from build123d import *

# Parameters (mm, degrees)
SKETCH1_R           = 0.575
SKETCH1_R_2         = 1.375
BOSS_EXTRUDE1_DEPTH = 1.2


with BuildPart() as part:
    # Sketch1 → Boss-Extrude1 (new body)
    with BuildSketch(Plane(origin=(0, 0, 0), x_dir=(1, 0, 0), z_dir=(0, 1, 0))):
        with BuildLine():
            Line((3, 0), (62, 0))
            ThreePointArc((62, 0), (64.121320344, 0.878679656), (65, 3))
            Line((65, 3), (65, 27))
            ThreePointArc((65, 27), (64.121320344, 29.121320344), (62, 30))
            Line((62, 30), (3, 30))
            ThreePointArc((3, 30), (0.878679656, 29.121320344), (0, 27))
            Line((0, 27), (0, 3))
            ThreePointArc((0, 3), (0.878679656, 0.878679656), (3, 0))
        make_face()
        with Locations((6.5, 27.85)):
            Circle(SKETCH1_R, mode=Mode.SUBTRACT)
        with Locations((9.236842105, 27.85)):
            Circle(SKETCH1_R, mode=Mode.SUBTRACT)
        with Locations((11.973684211, 27.85)):
            Circle(SKETCH1_R, mode=Mode.SUBTRACT)
        with Locations((14.710526316, 27.85)):
            Circle(SKETCH1_R, mode=Mode.SUBTRACT)
        with Locations((17.447368421, 27.85)):
            Circle(SKETCH1_R, mode=Mode.SUBTRACT)
        with Locations((20.184210526, 27.85)):
            Circle(SKETCH1_R, mode=Mode.SUBTRACT)
        with Locations((22.921052632, 27.85)):
            Circle(SKETCH1_R, mode=Mode.SUBTRACT)
        with Locations((25.657894737, 27.85)):
            Circle(SKETCH1_R, mode=Mode.SUBTRACT)
        with Locations((28.394736842, 27.85)):
            Circle(SKETCH1_R, mode=Mode.SUBTRACT)
        with Locations((31.131578947, 27.85)):
            Circle(SKETCH1_R, mode=Mode.SUBTRACT)
        with Locations((33.868421053, 27.85)):
            Circle(SKETCH1_R, mode=Mode.SUBTRACT)
        with Locations((36.605263158, 27.85)):
            Circle(SKETCH1_R, mode=Mode.SUBTRACT)
        with Locations((39.342105263, 27.85)):
            Circle(SKETCH1_R, mode=Mode.SUBTRACT)
        with Locations((42.078947368, 27.85)):
            Circle(SKETCH1_R, mode=Mode.SUBTRACT)
        with Locations((44.815789474, 27.85)):
            Circle(SKETCH1_R, mode=Mode.SUBTRACT)
        with Locations((47.552631579, 27.85)):
            Circle(SKETCH1_R, mode=Mode.SUBTRACT)
        with Locations((50.289473684, 27.85)):
            Circle(SKETCH1_R, mode=Mode.SUBTRACT)
        with Locations((53.026315789, 27.85)):
            Circle(SKETCH1_R, mode=Mode.SUBTRACT)
        with Locations((55.763157895, 27.85)):
            Circle(SKETCH1_R, mode=Mode.SUBTRACT)
        with Locations((58.5, 27.85)):
            Circle(SKETCH1_R, mode=Mode.SUBTRACT)
        with Locations((9.236842105, 25.1)):
            Circle(SKETCH1_R, mode=Mode.SUBTRACT)
        with Locations((11.973684211, 25.1)):
            Circle(SKETCH1_R, mode=Mode.SUBTRACT)
        with Locations((14.710526316, 25.1)):
            Circle(SKETCH1_R, mode=Mode.SUBTRACT)
        with Locations((17.447368421, 25.1)):
            Circle(SKETCH1_R, mode=Mode.SUBTRACT)
        with Locations((20.184210526, 25.1)):
            Circle(SKETCH1_R, mode=Mode.SUBTRACT)
        with Locations((22.921052632, 25.1)):
            Circle(SKETCH1_R, mode=Mode.SUBTRACT)
        with Locations((25.657894737, 25.1)):
            Circle(SKETCH1_R, mode=Mode.SUBTRACT)
        with Locations((28.394736842, 25.1)):
            Circle(SKETCH1_R, mode=Mode.SUBTRACT)
        with Locations((31.131578947, 25.1)):
            Circle(SKETCH1_R, mode=Mode.SUBTRACT)
        with Locations((33.868421053, 25.1)):
            Circle(SKETCH1_R, mode=Mode.SUBTRACT)
        with Locations((36.605263158, 25.1)):
            Circle(SKETCH1_R, mode=Mode.SUBTRACT)
        with Locations((39.342105263, 25.1)):
            Circle(SKETCH1_R, mode=Mode.SUBTRACT)
        with Locations((42.078947368, 25.1)):
            Circle(SKETCH1_R, mode=Mode.SUBTRACT)
        with Locations((44.815789474, 25.1)):
            Circle(SKETCH1_R, mode=Mode.SUBTRACT)
        with Locations((47.552631579, 25.1)):
            Circle(SKETCH1_R, mode=Mode.SUBTRACT)
        with Locations((50.289473684, 25.1)):
            Circle(SKETCH1_R, mode=Mode.SUBTRACT)
        with Locations((53.026315789, 25.1)):
            Circle(SKETCH1_R, mode=Mode.SUBTRACT)
        with Locations((55.763157895, 25.1)):
            Circle(SKETCH1_R, mode=Mode.SUBTRACT)
        with Locations((58.5, 25.1)):
            Circle(SKETCH1_R, mode=Mode.SUBTRACT)
        with Locations((6.5, 25.1)):
            Circle(SKETCH1_R, mode=Mode.SUBTRACT)
        with Locations((3.5, 26.5)):
            Circle(SKETCH1_R_2, mode=Mode.SUBTRACT)
        with Locations((61.5, 26.5)):
            Circle(SKETCH1_R_2, mode=Mode.SUBTRACT)
        with Locations((61.5, 3.5)):
            Circle(SKETCH1_R_2, mode=Mode.SUBTRACT)
        with Locations((3.5, 3.5)):
            Circle(SKETCH1_R_2, mode=Mode.SUBTRACT)
    extrude(amount=BOSS_EXTRUDE1_DEPTH)


solid = part.part
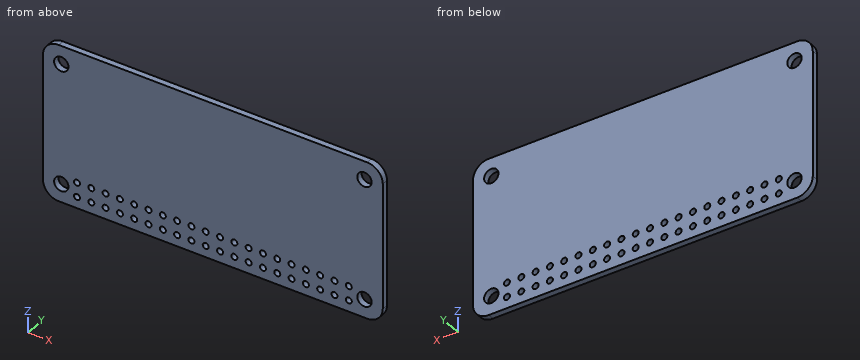
Source: CAD feature listing. Evaluate the final solid. Frame: model axes, mm. Round coordinates to 2 decimals unless told otherwise and drop trailing zeros. Loops run counter-clockwise (first coordinate to the right, second up) from the corner with the lowest first, then second, coordinate; pieces in that order, holes last.
Q1. Ray query, line 1 (Z direction, x = 58.5, y = 0.8) (3 decimals); line 2 (X direction, y = 0.35, z = -26.5) (3 decimals); line 3 (Z direction, x = 61.5, y = 0.85) (3 decimals). Return the intervals inside material, ascending.
Q2. Section A-A, the plane x = 6.5. Return loops of the section in (y, z) (3 decimals), plus the area to 3 significant figures.
Q3. Section B-B, the plane y = 0.85. State how many separate pieces and enclosed holes the cut face has, plus the area to 3 significant figures.
Solutions:
1. line 1: z = -30 to -28.425, -27.275 to -25.675, -24.525 to 0
1. line 2: x = 0 to 2.125, 4.875 to 60.125, 62.875 to 65
1. line 3: z = -30 to -27.875, -25.125 to -4.875, -2.125 to 0
2. outline: (0, -30) - (1.2, -30) - (1.2, -28.425) - (0, -28.425) - close; (0, -27.275) - (1.2, -27.275) - (1.2, -25.675) - (0, -25.675) - close; (0, -24.525) - (1.2, -24.525) - (1.2, 0) - (0, 0) - close
2. area: 33.2 mm2
3. separate pieces: 1
3. enclosed holes: 44
3. area: 1,880 mm2
